Here's how the part is built. I have some questions about the finished solid (model axes, mm). A direction names the side the tool comes from. Coordinates: 2 decimals unless noted, no trailing zeros. Loops run counter-clockwise (first coordinate to the right, second up) from the corner with the lowest first, then second, coordinate; pieces in that order, holes last. Notation, with made-up numbers: M 24,29 L 64,29 A20 cw 64,35 Z; hole C 46.5,18 d10. An arc over 180 degrees is marked long. Use CSV: the item, a comma, the result in double quotes. Start each with the question number.
Q1. If we section it at C-C (z = 1): Please give me the cut outline in (x, y).
Q2. For pin 1 Ø1 at (y, z) = (-2.5, 2) entering from -X; pin 2 Ø3.5 at (x, y) = (-1.5, 0) entering from +Z, each with a flat end and sliding along its axis, tell me the tip position at first contact or that it passes through.
Q3. Which directions (+Z, -Z, +X, -X, +Y, -Y) give clear straight access to the entire face, cutting with the end or side of a thin tool? Please do faces 4 (the flat face through (0, 0, 0.6)), 5 (the flat face through (0, 0, 0)).
Q4. Please list where these lines run through material, in increasing order: probe 1 along Y at (x, z) = (0, 3.5); probe 2 along Z at (x, y) = (1.5, -0.25); probe 3 along X at (y, z) = (-2.25, 5.25). Write a range as [from, to].
Q5. If we section it at A-A (x = 0): Please give me the cut outline in (y, z), and give its area (3 significant figures).
Q6. If we mould it in two halves opening along Y, with no side actions, what happens to faces 1 (the cylindrical face through (-0.74, -3.32, 4.25)), 2 (the cylindrical face through (2.58, 4.05, 3.85)), 3 (the flat face through (2, -3, 8))? For each: +Y half, -Y half, draft (parallel to the pull), parting line (faces both ways), or undercut.
from build123d import *

# Parameters (mm, degrees)
F0_R     = 3.4
F1_DEPTH = 0.6
F0_R_2   = 4.8
F2_DEPTH = 8
F3_SIZE  = 0.4
F4_SIZE  = 0.6


with BuildPart() as f1:
    # F0 (on Top) → F1 (new body)
    with BuildSketch(Plane.XY):
        Circle(F0_R)
    extrude(amount=F1_DEPTH)

    # F0 (on Top) → F2 (join)
    with BuildSketch(Plane.XY):
        Circle(F0_R_2)
        Circle(F0_R, mode=Mode.SUBTRACT)
    extrude(amount=F2_DEPTH)

    # F3
    f3_edges = [f1.edges().sort_by_distance(p)[0] for p in [
        (-4.8, 0, 0),
    ]]
    chamfer(f3_edges, length=F3_SIZE)

    # F4
    f4_edges = [f1.edges().sort_by_distance(p)[0] for p in [
        (-4.8, 0, 8),
    ]]
    chamfer(f4_edges, length=F4_SIZE)


solid = f1.part
Results below:
1,outline,"C 0,0 d9.6; hole C 0,0 d6.8"
2,pin 1,"x = -4.36"
2,pin 2,"z = 0.6"
3,face 4,"+Z"
3,face 5,"-Z, +X, -X, +Y, -Y"
4,probe 1,"[-4.8, -3.4], [3.4, 4.8]"
4,probe 2,"[0, 0.6]"
4,probe 3,"[-4.24, -2.55], [2.55, 4.24]"
5,outline,"M -4.8,0.4 L -4.4,0 L 4.4,0 L 4.8,0.4 L 4.8,7.4 L 4.2,8 L 3.4,8 L 3.4,0.6 L -3.4,0.6 L -3.4,8 L -4.2,8 L -4.8,7.4 Z"
5,area,"26.0 mm^2"
6,face 1,"undercut"
6,face 2,"parting line"
6,face 3,"draft"
